```python
from build123d import *

# Parameters (mm, degrees)
SKETCH3_W                     = 50.8
SKETCH3_H                     = 50.8
BOSS_EXTRUDE2_DEPTH           = 5.08
SKETCH4_R                     = 2.032
CUT_EXTRUDE2_DEPTH            = 73.021430144
FILLET2_R                     = 12.7
BOSS_EXTRUDE3_DEPTH           = 2.54
SKETCH6_R                     = 3.175
BOSS_EXTRUDE4_DEPTH           = 25.4
BOSS_EXTRUDE4_DRAFT           = 5
BOSS_EXTRUDE4_PROFILE_2_DEPTH = 25.4
BOSS_EXTRUDE4_PROFILE_2_DRAFT = 5
BOSS_EXTRUDE4_PROFILE_3_DEPTH = 25.4
BOSS_EXTRUDE4_PROFILE_3_DRAFT = 5
BOSS_EXTRUDE4_PROFILE_4_DEPTH = 25.4
BOSS_EXTRUDE4_PROFILE_4_DRAFT = 5
SKETCH7_R                     = 7.081764105
CUT_EXTRUDE3_DEPTH            = 201.795428329


with BuildPart() as part:
    # Sketch3 → Boss-Extrude2 (new body)
    with BuildSketch(Plane.XY):
        with Locations((25.4, 25.4)):
            Rectangle(SKETCH3_W, SKETCH3_H)
    extrude(amount=BOSS_EXTRUDE2_DEPTH)

    # Sketch4 → Cut-Extrude2 (cut, through all)
    with BuildSketch(Plane.XY.offset(5.08)):
        with Locations((12.7, 12.7)):
            Circle(SKETCH4_R)
    extrude(amount=-CUT_EXTRUDE2_DEPTH, mode=Mode.SUBTRACT)

    # Fillet2
    fillet2_edges = [part.edges().sort_by_distance(p)[0] for p in [
        (0, 50.8, 2.54),
        (50.8, 50.8, 2.54),
        (50.8, 0, 2.54),
        (0, 0, 2.54),
    ]]
    fillet(fillet2_edges, radius=FILLET2_R)

    # Sketch5 → Boss-Extrude3 (add)
    with BuildSketch(Plane.XY.offset(5.08)):
        Polygon((127.902561211, -89.802561211), (38.1, 0), (50.8, 12.7), (140.602561211, -77.102561211), align=None)
        Polygon((-89.802561211, -77.102561211), (0, 12.7), (12.7, 0), (-77.102561211, -89.802561211), align=None)
        Polygon((0, 38.1), (-89.802561211, 127.902561211), (-77.102561211, 140.602561211), (12.7, 50.8), align=None)
        Polygon((50.8, 38.1), (140.602561211, 127.902561211), (127.902561211, 140.602561211), (38.1, 50.8), align=None)
    extrude(amount=-BOSS_EXTRUDE3_DEPTH)


with BuildPart() as boss_extrude4_tool:
    # Sketch6 → Boss-Extrude4 (with draft: the straight prism first)
    with BuildSketch(Plane(origin=(0, 0, 2.54), x_dir=(-1, 0, 0), z_dir=(0, 0, -1))):
        with Locations((-129.76243315, 129.76243315)):
            Circle(SKETCH6_R)
    extrude(amount=BOSS_EXTRUDE4_DEPTH)
    # Boss-Extrude4: the draft: its side faces are tilted about the plane it starts from
    boss_extrude4_sides = [boss_extrude4_tool.faces().sort_by_distance(p)[0] for p in [
        (132.93743315, 129.76243315, -10.16),
    ]]
    draft(boss_extrude4_sides, Plane(origin=(0, 0, 2.54), x_dir=(-1, 0, 0), z_dir=(0, 0, -1)), BOSS_EXTRUDE4_DRAFT)


with BuildPart() as part_1:
    add(part.part)

    # Boss-Extrude4: add boss_extrude4_tool
    add(boss_extrude4_tool.part)


with BuildPart() as boss_extrude4_profile_2_tool:
    # Sketch6 → Boss-Extrude4 profile 2 (with draft: the straight prism first)
    with BuildSketch(Plane(origin=(0, 0, 2.54), x_dir=(-1, 0, 0), z_dir=(0, 0, -1))):
        with Locations((78.96243315, 129.76243315)):
            Circle(SKETCH6_R)
    extrude(amount=BOSS_EXTRUDE4_PROFILE_2_DEPTH)
    # Boss-Extrude4 profile 2: the draft: its side faces are tilted about the plane it starts from
    boss_extrude4_profile_2_sides = [boss_extrude4_profile_2_tool.faces().sort_by_distance(p)[0] for p in [
        (-75.78743315, 129.76243315, -10.16),
    ]]
    draft(boss_extrude4_profile_2_sides, Plane(origin=(0, 0, 2.54), x_dir=(-1, 0, 0), z_dir=(0, 0, -1)), BOSS_EXTRUDE4_PROFILE_2_DRAFT)


with BuildPart() as part_2:
    add(part_1.part)

    # Boss-Extrude4 profile 2: add boss_extrude4_profile_2_tool
    add(boss_extrude4_profile_2_tool.part)


with BuildPart() as boss_extrude4_profile_3_tool:
    # Sketch6 → Boss-Extrude4 profile 3 (with draft: the straight prism first)
    with BuildSketch(Plane(origin=(0, 0, 2.54), x_dir=(-1, 0, 0), z_dir=(0, 0, -1))):
        with Locations((78.96243315, -78.96243315)):
            Circle(SKETCH6_R)
    extrude(amount=BOSS_EXTRUDE4_PROFILE_3_DEPTH)
    # Boss-Extrude4 profile 3: the draft: its side faces are tilted about the plane it starts from
    boss_extrude4_profile_3_sides = [boss_extrude4_profile_3_tool.faces().sort_by_distance(p)[0] for p in [
        (-75.78743315, -78.96243315, -10.16),
    ]]
    draft(boss_extrude4_profile_3_sides, Plane(origin=(0, 0, 2.54), x_dir=(-1, 0, 0), z_dir=(0, 0, -1)), BOSS_EXTRUDE4_PROFILE_3_DRAFT)


with BuildPart() as part_3:
    add(part_2.part)

    # Boss-Extrude4 profile 3: add boss_extrude4_profile_3_tool
    add(boss_extrude4_profile_3_tool.part)


with BuildPart() as boss_extrude4_profile_4_tool:
    # Sketch6 → Boss-Extrude4 profile 4 (with draft: the straight prism first)
    with BuildSketch(Plane(origin=(0, 0, 2.54), x_dir=(-1, 0, 0), z_dir=(0, 0, -1))):
        with Locations((-129.76243315, -78.96243315)):
            Circle(SKETCH6_R)
    extrude(amount=BOSS_EXTRUDE4_PROFILE_4_DEPTH)
    # Boss-Extrude4 profile 4: the draft: its side faces are tilted about the plane it starts from
    boss_extrude4_profile_4_sides = [boss_extrude4_profile_4_tool.faces().sort_by_distance(p)[0] for p in [
        (132.93743315, -78.96243315, -10.16),
    ]]
    draft(boss_extrude4_profile_4_sides, Plane(origin=(0, 0, 2.54), x_dir=(-1, 0, 0), z_dir=(0, 0, -1)), BOSS_EXTRUDE4_PROFILE_4_DRAFT)


with BuildPart() as part_4:
    add(part_3.part)

    # Boss-Extrude4 profile 4: add boss_extrude4_profile_4_tool
    add(boss_extrude4_profile_4_tool.part)

    # Sketch7 → Cut-Extrude3 (cut, through all)
    with BuildSketch(Plane.XY.offset(5.08)):
        with Locations((30.660512242, 30.660512242)):
            Circle(SKETCH7_R)
    extrude(amount=-CUT_EXTRUDE3_DEPTH, mode=Mode.SUBTRACT)


solid = part_4.part
```
Geometry: final body of the model. Coordinates: model frame, mm. A direction names the side the tool comes from. Give positions to 0.01 mm unless a question says otherwise; leave off trailing zeros. Order: outer loops, then holes, each group sorted by start corner. A loop starts at its lowest first (then second) coordinate and runs counter-clockwise, first axis right, second up. Notation, with made-up numbers: (53, 71.5) -> (81, 71.5) arc R23 ccw to (81, 99.5) -> close; hole circle Ø7 at (89, 50.25). An arc over 180 degrees is marked (long way). Write each question's results on one line, items separated by ' | '. Start each with the question number.
1) Section C-C (z = -18.5). Return loops of the section in (x, y).
2) Set-up query: faces 1 (the flat face through (83.6, 96.3, 3.8)), 2 (the flat face through (50.8, 25, 3)), 3 (the flat face through (25, 0, 3)). Return all of +Z, -Z, +X, -X, +Y, -Y with unobstructed straight access to the full face (end or side cutting, diameter ignored); none if empty.
3) First-contact query: pin 1 (4 mm diameter, centred on y = 29.5, z = 3, fed in from -X); pin 2 (6.5 mm diameter, centred on x = 12.7, y = 12.7, fed in from +Z); pin 3 (5.5 mm diameter, centred on x = 29, z = 2, fed in from +Y); pin 4 (1.5 mm diameter, centred on x = 21, z = 2, fed in from -Y). Flat tips, straight axial feed; report the tip coordinate or a pass-through.
4) Section B-B (x = 97.5). Return loops of the section in (y, z), then the cut area to 3 significant figures.
5) Line query: line 1 (Y direction, x = 12.7, z = 2.2); line 2 (Z direction, x = -55, y = 99); line 3 (X direction, y = 68, z = 4.25). Output: solid intervals per line, ascending. Write a range as from..to.
6) Section D-D (z = -5). Return loops of the section in (x, y), then the cut area to 3 significant figures.
7) Section A-A (y = 61). Return loops of the section in (x, z).
8) Draft query along Y for faces 4 (the flat face through (25, 26, 0)), 5 (the conical face through (131.84, -78.87, -9.98)), 6 (the flat face through (-83.541, 134.164, 3.828)). Return one class per face: pulls with the +Y half, pulls with the -Y half, needs draft (parallel to the pull), parting line crosses it, or undercut.
Calculated:
1) outline: circle Ø2.67 at (-78.96, -78.96); circle Ø2.67 at (-78.96, 129.76); circle Ø2.67 at (129.76, -78.96); circle Ø2.67 at (129.76, 129.76)
2) face 1: +Z, -Z, +Y | face 2: +Z, -Z, +X | face 3: +Z, -Z, -Y
3) pin 1: x = 0 | pin 2: z = 5.08 | pin 3: y = 50.8 | pin 4: y = 0
4) outline: (-59.4, 2.54) -> (-34, 2.54) -> (-34, 5.08) -> (-59.4, 5.08) -> close; (84.8, 2.54) -> (110.2, 2.54) -> (110.2, 5.08) -> (84.8, 5.08) -> close | area: 129 mm2
5) line 1: 0..10.67, 14.73..50.8 | line 2: 2.54..5.08 | line 3: -29.9..-4.5, 55.3..80.7
6) outline: circle Ø5.03 at (-78.96, -78.96); circle Ø5.03 at (-78.96, 129.76); circle Ø5.03 at (129.76, -78.96); circle Ø5.03 at (129.76, 129.76) | area: 79.5 mm2
7) outline: (-22.9, 2.54) -> (2.5, 2.54) -> (2.5, 5.08) -> (-22.9, 5.08) -> close; (48.3, 2.54) -> (73.7, 2.54) -> (73.7, 5.08) -> (48.3, 5.08) -> close
8) face 4: needs draft | face 5: undercut | face 6: pulls with the +Y half
